Autodesk Fusion 360 part; units mm, degrees
sketch "Sketch1" plane through (0, 0, 0) normal (1, 0, 0) x (0, 0, -1)
  line L0 (-50.8576, -27.0879) -> (-50.8576, 45.2121)
  line L1 (62.6424, 47.2121) -> (-52.8576, 47.2121)
  line L2 (59.6424, 28.8121) -> (62.6424, 28.8121)
  line L3 (62.6424, 28.8121) -> (62.6424, 47.2121)
  line L4 (59.6424, 12.3121) -> (59.6424, -4.0879)
  line L5 (59.6424, 45.2121) -> (59.6424, 28.8121)
  line L6 (-50.8576, 45.2121) -> (59.6424, 45.2121)
  line L7 (17.6424, -6.0879) -> (62.6424, -6.0879)
  line L8 (59.6424, -4.0879) -> (5.6424, -4.0879)
  line L9 (62.6424, 12.3121) -> (59.6424, 12.3121)
  line L10 (-52.8576, 47.2121) -> (-52.8576, -29.0879)
  line L11 (-52.8576, -29.0879) -> (7.6424, -29.0879)
  line L12 (5.6424, -27.0879) -> (-50.8576, -27.0879)
  line L13 (5.6424, -4.0879) -> (5.6424, -27.0879)
  line L14 (7.6424, -29.0879) -> (7.6424, -16.0879)
  line L15 (62.6424, -6.0879) -> (62.6424, 12.3121)
  line L16 (59.6424, 28.8121) -> (59.6424, 12.3121)
  line L17 (62.6424, 12.3121) -> (62.6424, 28.8121)
  arc A0 (17.6424, -6.0879) -> (7.6424, -16.0879) centre (17.6424, -16.0879) ccw
  point P0 (62.6424, -13.1879)
  dimension "d9" = 10
extrude "Extrude1" add sketch "Sketch1" against normal blind 4 contours L0 L4 L5 L6 L8 L12 L13 L16
extrude "Extrude2" add sketch "Sketch1" against normal blind 2 contours L0 L1 L2 L3 L4 L5 L6 L7 L8 L9 L10 L11 L12 L13 L14 L15 A0
extrude "Extrude3" add sketch "Sketch1" against normal blind 40.55 contours L2 L9 L16 L17
sketch "Sketch3" plane through (0, 0, 0) normal (1, 0, 0) x (0, 0, -1)
  line L0 (62.6424, -6.0879) -> (62.6424, 47.2121)
  line L1 (62.6424, 47.2121) -> (-52.8576, 47.2121)
  line L2 (-52.8576, 47.2121) -> (-52.8576, -29.0879)
  line L3 (-52.8576, -29.0879) -> (7.6424, -29.0879)
  line L4 (7.6424, -29.0879) -> (7.6424, -16.0879)
  arc A0 (17.6424, -6.0879) -> (7.6424, -16.0879) centre (17.6424, -16.0879) ccw
  line L5 (17.6424, -6.0879) -> (62.6424, -6.0879)
  circle A1 centre (8.5297, -6.9752) radius 1.75
  line L6 (5.6424, -4.0879) -> (5.6424, -27.0879) construction
  line L7 (59.6424, -4.0879) -> (5.6424, -4.0879) construction
  line L8 (8.5297, -5.2252) -> (8.5297, -4.0879) construction
  line L9 (6.7797, -6.9752) -> (5.6424, -6.9752) construction
  line L10 (9.7672, -8.2126) -> (10.5714, -9.0168) construction
  point P0 (5.6424, -4.0879)
  dimension "d10" = 3.5
extrude "Extrude4" cut sketch "Sketch3" against normal blind 2 contours A1
Part model, mm, in its own coordinate system. A direction names the side the tool comes from. Coordinates: 2 decimals unless noted, no trailing zeros. Loops run counter-clockwise (first coordinate to the right, second up) from the corner with the lowest first, then second, coordinate; pieces in that order, holes last. Notation, with made-up numbers: (77, 63.5) -> (123, 63.5) arc R23 ccw to (123, 71.5) -> close; hole circle Ø9 at (-16.75, 2). An arc over 180 degrees is marked (long way). Use a Markdown table: item, result. Add a question column.
Item 1: Band-saw the part on A-A on y = -22. Write the cut outline in (x, z).
Item 2: Band-saw the part on C-C on x = -26. Write the cut outline in (y, z).
Item 3: Flat gauge pins, fed straight in: P1, Ø2.5, axis at x = -14.5, z = -61, coming from the -Y side; P2, Ø21.5, axis at y = -6, z = 17.5, coming from the -X side; P3, Ø2, axis at x = -0.5, y = -22.5, coming from the -Z side; P4, Ø6, axis at x = -8, y = 9, coming from the +Z side. Where does each tip first touch, or does it go through?
Item 4: Probe probe 1 along X at (y, z) = (-18.5, -3); probe 2 along Y at (x, z) = (-3, -15.5); probe 3 along Z at (x, y) = (-30, 14.5). List the from-to ranges inside material, lowest first.
Item 5: Band-saw the part on B-B on z = 2.5. Write the cut outline in (x, y).
Item 6: Which spindle directions (+Z, -Z, +X, -X, +Y, -Y) get a long thin tool onto all of the face, cutting with end or side? Do faces 1 (the flat face through (-15, 20, -62.642)), 2 (the flat face through (-4, 18, -4)). Say none if no direction does.
Geometry says:
| question | item | result |
|---|---|---|
| 1 | outline | (-4, -5.64) -> (-2, -5.64) -> (-2, -7.64) -> (0, -7.64) -> (0, 52.86) -> (-2, 52.86) -> (-2, 50.86) -> (-4, 50.86) -> close |
| 2 | outline | (12.31, -62.64) -> (28.81, -62.64) -> (28.81, -59.64) -> (12.31, -59.64) -> close |
| 3 | P1 | y = 12.31 |
| 3 | P2 | x = -4 |
| 3 | P3 | z = -7.64 |
| 3 | P4 | through |
| 4 | probe 1 | -4 to 0 |
| 4 | probe 2 | -4.09 to 45.21 |
| 4 | probe 3 | -62.64 to -59.64 |
| 5 | outline | (-4, -27.09) -> (-2, -27.09) -> (-2, -29.09) -> (0, -29.09) -> (0, 47.21) -> (-2, 47.21) -> (-2, 45.21) -> (-4, 45.21) -> close |
| 6 | face 1 | -Z, +X, -X, +Y, -Y |
| 6 | face 2 | +Z, -X, +Y, -Y |
